```python
from build123d import *

# Parameters (mm, degrees)
BOSS_EXTRUDE1_DEPTH   = 2.5
BOSS_EXTRUDE1_2_DEPTH = 2.5
BOSS_EXTRUDE1_3_DEPTH = 2.5
SKETCH1_3_R           = 40
SKETCH1_3_R_2         = 25
BOSS_EXTRUDE2_DEPTH   = 5


with BuildPart() as part:
    # Sketch1 → Boss-Extrude1 (new, symmetric)
    with BuildSketch(Plane.XY):
        with BuildLine():
            Line((-40.593283957, 10.704662693), (42.324676718, 58.57736961))
            ThreePointArc((42.324676718, 58.57736961), (36.224680229, 66.602540378), (32.324676718, 75.897877685))
            Line((32.324676718, 75.897877685), (-50.593283957, 28.025170769))
            ThreePointArc((-50.593283957, 28.025170769), (-44.493287469, 20), (-40.593283957, 10.704662693))
        make_face()
    extrude(amount=BOSS_EXTRUDE1_DEPTH, both=True)



with BuildPart() as body_2:
    # Sketch1 → Boss-Extrude1 2 (new, symmetric)
    with BuildSketch(Plane.XY):
        with BuildLine():
            ThreePointArc((32.324540751, -75.895826853), (36.224426192, -66.600440011), (42.324320743, -58.575191763))
            Line((42.324320743, -58.575191763), (-40.593147991, -10.704173147))
            ThreePointArc((-40.593147991, -10.704173147), (-44.493033432, -19.999559989), (-50.592927983, -28.024808237))
            Line((-50.592927983, -28.024808237), (32.324540751, -75.895826853))
        make_face()
    extrude(amount=BOSS_EXTRUDE1_2_DEPTH, both=True)


with BuildPart() as body_3:
    # Sketch1 → Boss-Extrude1 3 (new, symmetric)
    with BuildSketch(Plane.XY):
        with BuildLine():
            ThreePointArc((80.86569638, 47.872706916), (70.86569638, 46.602540378), (60.86569638, 47.872706916))
            Line((60.86569638, 47.872706916), (60.86569638, -47.870166538))
            ThreePointArc((60.86569638, -47.870166538), (70.86569638, -46.6), (80.86569638, -47.870166538))
            Line((80.86569638, -47.870166538), (80.86569638, 47.872706916))
        make_face()
    extrude(amount=BOSS_EXTRUDE1_3_DEPTH, both=True)


with BuildPart() as part_1:
    add(part.part)

    add(body_2.part)  # Boss-Extrude2 merges body 2

    add(body_3.part)  # Boss-Extrude2 merges body 3
    # Sketch1<3> → Boss-Extrude2 (add, symmetric)
    # profile 1 of 3: a face of its own
    with BuildSketch(Plane.XY):
        with Locations((-79.13430362, 0)):
            Circle(SKETCH1_3_R)
        with Locations((-79.13430362, 0)):
            Circle(SKETCH1_3_R_2, mode=Mode.SUBTRACT)
    # profile 2 of 3: a face of its own
    with BuildSketch(Plane.XY):
        with Locations((70.86569638, 86.602540378)):
            Circle(SKETCH1_3_R)
        with Locations((70.86569638, 86.602540378)):
            Circle(SKETCH1_3_R_2, mode=Mode.SUBTRACT)
    # profile 3 of 3: a face of its own
    with BuildSketch(Plane.XY):
        with Locations((70.86569638, -86.6)):
            Circle(SKETCH1_3_R)
        with Locations((70.86569638, -86.6)):
            Circle(SKETCH1_3_R_2, mode=Mode.SUBTRACT)
    extrude(amount=BOSS_EXTRUDE2_DEPTH, both=True)


solid = part_1.part
```
Part model, mm, in its own coordinate system. A direction names the side the tool comes from. Give positions to 0.01 mm unless a question says otherwise; leave off trailing zeros. Order: outer loops, then holes, each group sorted by start corner. A loop starts at its lowest first (then second) coordinate and runs counter-clockwise, first axis right, second up. Notation, with made-up numbers: (70, -17.5) - (124, -17.5) arc R20 ccw to (124, 6.5) - close; hole circle Ø1 at (29.25, 55.5). An arc over 180 degrees is marked (long way). Use one line per item in the form item = value.
Item 1: Which spindle directions (+Z, -Z, +X, -X, +Y, -Y) get a long thin tool onto all of the face, cutting with end or side? Do faces 3 (the face through (0.29, 34.31, 0.04)), 4 (the face through (88.08, 104.94, -5)). Say none if no direction does.
Solution:
face_3 = +Z, -Z
face_4 = -Z, +X, -X, +Y, -Y
Item 2: Slice it at B-B on y = 0. Give the cut face in (x, z).
Solution:
outline = (-119.13, -5) - (-104.13, -5) - (-104.13, 5) - (-119.13, 5) - close; (-54.13, -5) - (-39.13, -5) - (-39.13, 5) - (-54.13, 5) - close; (60.87, -2.5) - (80.87, -2.5) - (80.87, 2.5) - (60.87, 2.5) - close
Item 3: Slice it at C-C on x = 3.5. Give the cut face in (y, z).
Solution:
outline = (-59.25, -2.5) - (-36.16, -2.5) - (-36.16, 2.5) - (-59.25, 2.5) - close; (36.16, -2.5) - (59.26, -2.5) - (59.26, 2.5) - (36.16, 2.5) - close
Item 4: Slice it at D-D on z = -0.75. Give the cut face in (x, y), and give its area (3 significant figures).
Solution:
outline = (-50.59, -28.02) - (32.32, -75.9) arc R40 ccw (long way) to (80.87, -47.87) - (80.87, 47.87) arc R40 ccw (long way) to (32.32, 75.9) - (-50.59, 28.03) arc R40 ccw (long way) to start; hole circle Ø50 at (-79.13, 0); hole (-40.59, -10.7) - (42.32, -58.58) arc R40 cw to (60.87, -47.87) - (60.87, 47.87) arc R40 cw to (42.32, 58.58) - (-40.59, 10.7) arc R40 cw to start; hole circle Ø50 at (70.87, -86.6); hole circle Ø50 at (70.87, 86.6)
area = 14,800 mm2
Item 5: Pin check, flat tips, straight feed: pin 1 Ø1 at (x, z) = (58.5, 1) entering from -Y; pin 2 Ø1.5 at (y, z) = (-10.5, 0) entering from +X; pin 3 Ø10 at (x, y) = (67.5, -21.5) entering from -Z. Stop position of each tip, or through.
Solution:
pin_1 = -124.8
pin_2 = 80.87
pin_3 = -2.5
Item 6: Two-plate mould, pull along Y, no slides. Class faces 1 (the face through (52.5, -103.8, 5)), 2 (the face through (89.3, -122.1, 0.1)): released by +Y, released by -Y, zero draft, split by the parting line, or undercut.
Solution:
face_1 = zero draft
face_2 = undercut
Item 7: Probe probe 1 along X at (y, z) = (-0.5, 1.75); probe 2 along Y at (x, z) = (-79, -0.5); probe 3 along Y at (x, z) = (54.5, 0.75). List the from-to ranges inside material, lowest first. Write a range as from..to.
Solution:
probe_1 = -119.13..-104.13, -54.14..-39.14, 60.87..80.87
probe_2 = -40..-25, 25..40
probe_3 = -123.1..-105.5, -67.7..-50.1, 50.1..67.7, 105.5..123.1
Item 8: Slice it at A-A on y = -86.6. Give the cut face in (x, z), and give its area (3 significant figures).
Solution:
outline = (30.87, -5) - (45.87, -5) - (45.87, 5) - (30.87, 5) - close; (95.87, -5) - (110.87, -5) - (110.87, 5) - (95.87, 5) - close
area = 300 mm2
